from build123d import *

# Parameters (mm, degrees)
SKETCH_1_W          = 20
SKETCH_1_H          = 50
SKETCH_1_W_2        = 16
SKETCH_1_H_2        = 40
EXTRUDE_1_DEPTH     = 700
SKETCH_5_R          = 2.1
CUT_EXTRUDE_1_DEPTH = 701.731760376
SKETCH_6_R          = 2
CUT_EXTRUDE_3_DEPTH = 702.854685815
SKETCH_7_R          = 2
CUT_EXTRUDE_5_DEPTH = 701.731760376


with BuildPart() as part:
    # 草图1 → 凸台-拉伸1 (new body)
    with BuildSketch(Plane.XY):
        Rectangle(SKETCH_1_W, SKETCH_1_H)
        Rectangle(SKETCH_1_W_2, SKETCH_1_H_2, mode=Mode.SUBTRACT)
    extrude(amount=EXTRUDE_1_DEPTH)

    # 草图5 → 切除-拉伸1 (cut, through all)
    with BuildSketch(Plane.ZY.offset(10)):
        with Locations((10, 10)):
            Circle(SKETCH_5_R)
        with Locations((20, 10)):
            Circle(SKETCH_5_R)
        with Locations((10, -10)):
            Circle(SKETCH_5_R)
        with Locations((20, -10)):
            Circle(SKETCH_5_R)
    cut_extrude_1 = extrude(amount=-CUT_EXTRUDE_1_DEPTH, mode=Mode.SUBTRACT)

    # 镜向1: 切除-拉伸1 across plane
    add(cut_extrude_1.mirror(Plane(origin=(-40, 280, 350), x_dir=(1, 0, 0), z_dir=(0, 0, -1))), mode=Mode.SUBTRACT)

    # 草图6 → 切除-拉伸3 (cut, through all)
    with BuildSketch(Plane.XZ.offset(25)):
        with Locations(Location((-3.5, 132, 0), (0, 0, 270))):
            Circle(SKETCH_6_R)
        with Locations(Location((4.5, 132, 0), (0, 0, 270))):
            Circle(SKETCH_6_R)
        with Locations(Location((4.5, 140, 0), (0, 0, 270))):
            Circle(SKETCH_6_R)
        with Locations(Location((4.5, 148, 0), (0, 0, 270))):
            Circle(SKETCH_6_R)
        with Locations(Location((4.5, 156, 0), (0, 0, 270))):
            Circle(SKETCH_6_R)
        with Locations(Location((4.5, 164, 0), (0, 0, 270))):
            Circle(SKETCH_6_R)
        with Locations(Location((-3.5, 140, 0), (0, 0, 270))):
            Circle(SKETCH_6_R)
        with Locations(Location((-3.5, 148, 0), (0, 0, 270))):
            Circle(SKETCH_6_R)
        with Locations(Location((-3.5, 156, 0), (0, 0, 270))):
            Circle(SKETCH_6_R)
        with Locations(Location((-3.5, 164, 0), (0, 0, 270))):
            Circle(SKETCH_6_R)
    extrude(amount=-CUT_EXTRUDE_3_DEPTH, mode=Mode.SUBTRACT)

    # 草图7 → 切除-拉伸5 (cut, through all)
    with BuildSketch(Plane.ZY.offset(10)):
        with Locations((600, 15)):
            Circle(SKETCH_7_R)
        with Locations((592, 15)):
            Circle(SKETCH_7_R)
        with Locations((584, 15)):
            Circle(SKETCH_7_R)
        with Locations((576, 15)):
            Circle(SKETCH_7_R)
        with Locations((568, 15)):
            Circle(SKETCH_7_R)
        with Locations(Location((592, -15, 0), (0, 0, 180))):
            Circle(SKETCH_7_R)
        with Locations(Location((584, -15, 0), (0, 0, 180))):
            Circle(SKETCH_7_R)
        with Locations(Location((576, -15, 0), (0, 0, 180))):
            Circle(SKETCH_7_R)
        with Locations(Location((568, -15, 0), (0, 0, 180))):
            Circle(SKETCH_7_R)
        with Locations(Location((600, -15, 0), (0, 0, 180))):
            Circle(SKETCH_7_R)
    extrude(amount=-CUT_EXTRUDE_5_DEPTH, mode=Mode.SUBTRACT)


solid = part.part
Work out the finished part from the listing and answer in its coordinate system (mm). A direction names the side the tool comes from. Give positions to 0.01 mm unless a question says otherwise; leave off trailing zeros. Write each loop counter-clockwise with the first axis right and the second up, starting at its lowest first coordinate (ties: lowest second). Pieces come first, ordered by that corner, then holes. Notation, with made-up numbers: (9, 59) - (18, 59) arc R28 ccw to (18, 97) - close; hole circle Ø9 at (87, 72). An arc over 180 degrees is marked (long way). One line per item, written item: value. Start each with the question number.
1. Find section B-B (z = 427.5). Write down the section's boundary in (x, y), then the cut area to 3 significant figures.
2. For faces 1 (the flat face through (8, 0, 345)), 2 (the flat face through (-9, 0, 700)), determine the directions among +Z, -Z, +X, -X, +Y, -Y from which every point of the face is accessible in a straight line to the end or side of a thin tool.
3. Consider probe 1 along Z at (x, y) = (8.8, -15); probe 2 along X at (y, z) = (-22, 140); probe 3 along Y at (x, z) = (8.6, 568). Determine where each line is inside the solid, lowest interval first.
4. Find section A-A (y = -0.5). Write down the section's boundary in (x, z), then the cut area to 3 significant figures.
5. For a pull along Y with two mould halves and no side action, classify faces 3 (the flat face through (0, -25, 345)), 4 (the flat face through (-8, 0, 345)), 5 (the flat face through (0, 25, 345)) as +Y half, -Y half, draft (parallel to the pull), parting line (faces both ways), or undercut.
Geometry results:
1. outline: (-10, -25) - (10, -25) - (10, 25) - (-10, 25) - close; hole (-8, -20) - (8, -20) - (8, 20) - (-8, 20) - close
1. area: 360 mm2
2. face 1: +Z, -Z
2. face 2: +Z, +X, -X, +Y, -Y
3. probe 1: 0 to 566, 570 to 574, 578 to 582, 586 to 590, 594 to 598, 602 to 700
3. probe 2: -10 to -5.5, -1.5 to 2.5, 6.5 to 10
3. probe 3: -25 to -17, -13 to 13, 17 to 25
4. outline: (-10, 0) - (-8, 0) - (-8, 700) - (-10, 700) - close; (8, 0) - (10, 0) - (10, 700) - (8, 700) - close
4. area: 2,800 mm2
5. face 3: -Y half
5. face 4: undercut
5. face 5: +Y half
